Could you check a few things on this model? Use its own coordinates, in mm. A direction names the side the tool comes from. Give positions to 0.01 mm unless a question says otherwise; leave off trailing zeros. Write each loop counter-clockwise with the first axis right and the second up, starting at its lowest first coordinate (ties: lowest second). Pieces come first, ordered by that corner, then holes. Notation, with made-up numbers: (52.25, 44.5) - (71.25, 44.5) arc R20 ccw to (71.25, 55.5) - close; hole circle Ø4 at (-20.5, -2). An arc over 180 degrees is marked (long way). Answer as CSV lines item,"result". Start each with the question number.
Q1. Imagine slicing it at B-B on x = 8. List the corners of the cut face in (y, z) for me.
Q2. Imagine slicing it at A-A on y = 8. List the corners of the cut face in (x, z) for me.
Q3. Imagine slicing it at C-C on z = 10. List the corners of the cut face in (x, y) for me, and give its area (3 significant figures).
Q4. Imagine slicing it at D-D on x = 80. List the corners of the cut face in (y, z) for me, and give its area (3 significant figures).
Q5. On a 3-axis mill with a long thin cutter (end or side, diameter ignored), from which of +Z, -Z, +X, -X, +Y, -Y can I reach the whole of each face in a straight line? I mean faces 1 (the face through (110, 30, 6)), 2 (the face through (3, 30, 9)). Say none if no direction works.
Q6. If I drill on line 1 along Y through (x, z) = (45.5, 10.75); line 2 along X through (y, z) = (13, 10.25); line 3 along Y through (x, z) = (8, 3.25), over which ranges is the centre line in solid material (lowest first)?
Q7. Will this pin go through, and if not, where does the flat tip stop? pin 1 Ø4 at (x, y) = (26, 14) entering from +Z.
Q8. We'd pull the mould along X, two halves only. Please class faces 3 (the face through (0, 30, 6)), 4 (the face through (54, 58, 9)), 5 (the face through (107, 30, 9)), 6 (the face through (54, 61, 6)): pulls with the +X half, pulls with the -X half, needs draft (parallel to the pull), parting line crosses it, or undercut.
```python
from build123d import *

# Parameters (mm, degrees)
SKETCH1_W           = 110
SKETCH1_H           = 61
BOSS_EXTRUDE1_DEPTH = 6.35
SKETCH3_W           = 110
SKETCH3_H           = 61
SKETCH3_W_2         = 104
SKETCH3_H_2         = 55
BOSS_EXTRUDE2_DEPTH = 6
SKETCH5_R           = 3
CUT_EXTRUDE1_DEPTH  = 126.941742484


with BuildPart() as part:
    # Sketch1 → Boss-Extrude1 (new body)
    with BuildSketch(Plane.XY):
        with Locations((55, 30.5)):
            Rectangle(SKETCH1_W, SKETCH1_H)
    extrude(amount=BOSS_EXTRUDE1_DEPTH)

    # Sketch3 → Boss-Extrude2 (add)
    with BuildSketch(Plane.XY.offset(6.35)):
        with Locations((55, 30.5)):
            Rectangle(SKETCH3_W, SKETCH3_H)
        with Locations((55, 30.5)):
            Rectangle(SKETCH3_W_2, SKETCH3_H_2, mode=Mode.SUBTRACT)
    extrude(amount=BOSS_EXTRUDE2_DEPTH)

    # Sketch5 → Cut-Extrude1 (cut, through all)
    with BuildSketch(Plane.XY.offset(6.35)):
        with Locations((8, 8)):
            Circle(SKETCH5_R)
    extrude(amount=-CUT_EXTRUDE1_DEPTH, mode=Mode.SUBTRACT)


solid = part.part
```
Conclusion:
1,outline,"(0, 0) - (5, 0) - (5, 6.35) - (3, 6.35) - (3, 12.35) - (0, 12.35) - close; (11, 0) - (61, 0) - (61, 12.35) - (58, 12.35) - (58, 6.35) - (11, 6.35) - close"
2,outline,"(0, 0) - (5, 0) - (5, 6.35) - (3, 6.35) - (3, 12.35) - (0, 12.35) - close; (11, 0) - (110, 0) - (110, 12.35) - (107, 12.35) - (107, 6.35) - (11, 6.35) - close"
3,outline,"(0, 0) - (110, 0) - (110, 61) - (0, 61) - close; hole (3, 3) - (107, 3) - (107, 58) - (3, 58) - close"
3,area,"990 mm^2"
4,outline,"(0, 0) - (61, 0) - (61, 12.35) - (58, 12.35) - (58, 6.35) - (3, 6.35) - (3, 12.35) - (0, 12.35) - close"
4,area,"423 mm^2"
5,face 1,"+Z, -Z, +X, +Y, -Y"
5,face 2,"+Z"
6,line 1,"0 to 3, 58 to 61"
6,line 2,"0 to 3, 107 to 110"
6,line 3,"0 to 5, 11 to 61"
7,pin 1,"z = 6.35"
8,face 3,"pulls with the -X half"
8,face 4,"undercut"
8,face 5,"undercut"
8,face 6,"needs draft"
